The listing builds one solid part. Answer for the finished solid, in the listing's coordinates (mm). Face numbers are marked on the shaded views. A direction names the side the tool comes from. Round coordinates to 2 decimals unless told otherwise and drop trailing zeros. Loops run counter-clockwise (first coordinate to the right, second up) from the corner with the lowest first, then second, coordinate; pieces in that order, holes last. Notation, with made-up numbers: (24, -30) - (54, -30) arc R15 ccw to (54, -12) - close; hole circle Ø1 at (18.25, 60.25). An arc over 180 degrees is marked (long way). One line per item, written item: value.
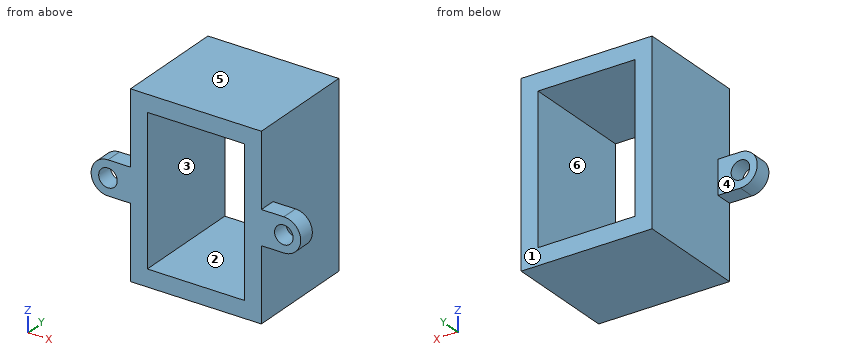
```python
from build123d import *

# Parameters (mm, degrees)
SKETCH1_W           = 23.3
SKETCH1_H           = 32
SKETCH1_W_2         = 17.3
SKETCH1_H_2         = 26
BOSS_EXTRUDE1_DEPTH = 20
SKETCH3_R           = 1.65
BOSS_EXTRUDE2_DEPTH = 3


with BuildPart() as part:
    # Sketch1 → Boss-Extrude1 (new body)
    with BuildSketch(Plane(origin=(0, 0, 0), x_dir=(1, 0, 0), z_dir=(0, 1, 0))):
        Rectangle(SKETCH1_W, SKETCH1_H)
        Rectangle(SKETCH1_W_2, SKETCH1_H_2, mode=Mode.SUBTRACT)
    extrude(amount=BOSS_EXTRUDE1_DEPTH)

    # Sketch3 → Boss-Extrude2 (add)
    with BuildSketch(Plane(origin=(0, 0, 0), x_dir=(1, 0, 0), z_dir=(0, 1, 0))):
        with BuildLine():
            Line((11.65, 3), (15.65, 3))
            ThreePointArc((15.65, 3), (18.65, 0), (15.65, -3))
            Line((15.65, -3), (11.65, -3))
            Line((11.65, -3), (11.65, 3))
        make_face()
        with Locations((15.65, 0)):
            Circle(SKETCH3_R, mode=Mode.SUBTRACT)
        with BuildLine():
            Line((-11.65, -3), (-15.65, -3))
            ThreePointArc((-15.65, -3), (-18.65, 0), (-15.65, 3))
            Line((-15.65, 3), (-11.65, 3))
            Line((-11.65, 3), (-11.65, -3))
        make_face()
        with Locations((-15.65, 0)):
            Circle(SKETCH3_R, mode=Mode.SUBTRACT)
    extrude(amount=BOSS_EXTRUDE2_DEPTH)


solid = part.part
```
1) For a pull along X with two mould halves and no side action, classify the marked faces 1, 2 and 3 as released by +X, released by -X, zero draft, split by the parting line, or undercut.
Final values:
face 1: zero draft
face 2: undercut
face 3: undercut
2) For the marked faces 4, 5 and 6, determine the directions among +Z, -Z, +X, -X, +Y, -Y from which every point of the face is accessible in a straight line to the end or side of a thin tool.
Final values:
face 4: +Z, -Z, -X, +Y
face 5: +Z, +X, -X, +Y, -Y
face 6: +Y, -Y
3) A cutting plane is placed at A-A on z = 0. Give the vertices of the cut face in (x, y).
Final values:
outline: (-18.65, 0) - (-17.3, 0) - (-17.3, 3) - (-18.65, 3) - close; (-14, 0) - (-8.65, 0) - (-8.65, 20) - (-11.65, 20) - (-11.65, 3) - (-14, 3) - close; (8.65, 0) - (14, 0) - (14, 3) - (11.65, 3) - (11.65, 20) - (8.65, 20) - close; (17.3, 0) - (18.65, 0) - (18.65, 3) - (17.3, 3) - close
4) A cutting plane is placed at C-C on x = 7. Give the vertices of the cut face in (y, z).
Final values:
outline: (0, -16) - (20, -16) - (20, -13) - (0, -13) - close; (0, 13) - (20, 13) - (20, 16) - (0, 16) - close
5) A cutting plane is placed at B-B on z = 9. Give the vertices of the cut face in (x, y).
Final values:
outline: (-11.65, 0) - (-8.65, 0) - (-8.65, 20) - (-11.65, 20) - close; (8.65, 0) - (11.65, 0) - (11.65, 20) - (8.65, 20) - close
6) Each of these flat-tipped pins is pushed along its axis until it touches: pin 1 Ø2.5 at (x, y) = (-14.5, 1) entering from +Z; pin 2 Ø1.5 at (x, y) = (-13.5, 1) entering from -Z; pin 3 Ø6 at (y, z) = (11, -3.5) entering from -X; pin 4 Ø1 at (x, z) = (-6.5, 4.5) entering from -Y. Where does it stop, or does it pass through?
Final values:
pin 1: z = 3
pin 2: z = -3
pin 3: x = -11.65
pin 4: through
7) A cutting plane is placed at D-D on y = 14. Give the vertices of the cut face in (x, z).
Final values:
outline: (-11.65, -16) - (11.65, -16) - (11.65, 16) - (-11.65, 16) - close; hole (-8.65, -13) - (8.65, -13) - (8.65, 13) - (-8.65, 13) - close
8) Consider L1, parallel to X at y = 0.9, z = 0; L2, parallel to X at y = 3.5, z = -2.5; L3, parallel to Z at x = -15.65, y = 0.85. Determine where each line is inside the solid, lowest interval first.
Final values:
L1: -18.65 to -17.3, -14 to -8.65, 8.65 to 14, 17.3 to 18.65
L2: -11.65 to -8.65, 8.65 to 11.65
L3: -3 to -1.65, 1.65 to 3
